```python
from build123d import *

# Parameters (mm, degrees)
F1_DEPTH = 12.7
F2_SIZE  = 6.34999
F4_D     = 22


# Not quite as in the source:
# - a fillet or chamfer is up to 0.001 mm smaller than in the source, because OpenCascade refuses the exact size


with BuildPart() as f1:
    # F0 (on Right) → F1 (new body)
    with BuildSketch(Plane.YZ):
        Polygon((0, 56.2922134995), (-25.5191382021, 25.3690239042), (-54.6409785748, 0), (-25.5191382021, -25.6692506373), (0, -56.8926632404), (25.2189133316, -25.6692506373), (54.9412034452, 0), (25.5191363394, 24.768576026), align=None)
    extrude(amount=F1_DEPTH)

    # F2 (size 6.35 in the source; OpenCascade refuses exactly that, so slightly less here)
    f2_edges = [f1.edges().sort_by_distance(p)[0] for p in [
        (12.7, -40.080058, 12.684512),
        (0, -40.080058, 12.684512),
        (12.7, -40.080058, -12.834625),
        (0, -40.080058, -12.834625),
        (12.7, -12.759569, -41.280957),
        (0, -12.759569, -41.280957),
        (0, 12.609457, -41.280957),
        (12.7, 12.609457, -41.280957),
        (0, 40.080058, -12.834625),
        (12.7, 40.080058, -12.834625),
        (12.7, 40.23017, 12.384288),
        (0, 40.23017, 12.384288),
        (0, 12.759568, 40.530395),
        (12.7, 12.759568, 40.530395),
        (0, -12.759569, 40.830619),
        (12.7, -12.759569, 40.830619),
    ]]
    chamfer(f2_edges, length=F2_SIZE)

    # F4 (through all)
    with Locations(Plane(origin=(0, 0, 0), x_dir=(0, 1, 0), z_dir=(-1, 0, 0))):
        with Locations((0, 0)):
            Hole(F4_D / 2)


solid = f1.part
```
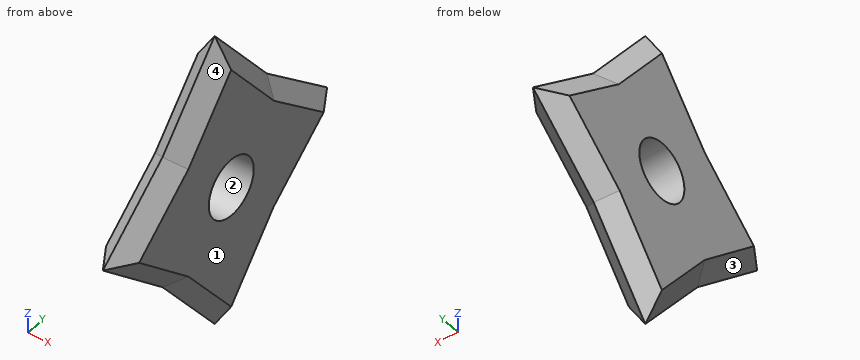
Part model, mm, in its own coordinate system. Face numbers are marked on the shaded views. Round coordinates to 2 decimals unless told otherwise and drop trailing zeros. Write each loop counter-clockwise with the first axis right and the second up, starting at its lowest first coordinate (ties: lowest second). Pieces come first, ordered by that corner, then holes. Notation, with made-up numbers: (-27.75, -2) -> (14.25, -2) arc R22 cw to (14.25, 35) -> close; hole circle Ø1 at (-29.5, 45.5). An arc over 180 degrees is marked (long way). Return JSON: item names as keys, results as strings. Group by question number.
Q1. Saw through at C-C on x = 1.75. Write the cut outline in (y, z), plus the area to 3 significant figures.
Q2. Mould opens along Z. For the marked faces 1, 2, 3 and 4 say: pulls with the +Z half, pulls with the -Z half, needs draft (parallel to the pull), parting line crosses it, or undercut.
Q3. Probe L1, parallel to Y at x = 9.5, z = -6; L2, parallel to Z at x = 6.5, y = 5; L3, parallel to Y at x = 1.25, z = -6. List the from-to ranges inside material, lowest first. Write a range as [from, to].
Q4. Pin check, flat tips, straight feed: pin 1 (1.5 mm diameter, centred on x = 3, y = -0.5, fed in from -Z); pin 2 (13 mm diameter, centred on y = 0, z = 0, fed in from +X); pin 3 (3 mm diameter, centred on x = 10, y = -25.5, fed in from +Z); pin 4 (6 mm diameter, centred on x = 10.5, y = 5.5, fed in from -Z). Stop position of each tip, or through.
Answer:
{
 "1": {"outline": "(-47.66, -0.02) -> (-22.2, -22.47) -> (-0.02, -49.6) -> (21.9, -22.46) -> (47.85, -0.04) -> (22.22, 21.53) -> (-0.03, 49.02) -> (-22.21, 22.15) -> close; hole circle Ø22 at (0, 0)", "area": "3,920 mm2"},
 "2": {"face 1": "needs draft", "face 2": "undercut", "face 3": "pulls with the -Z half", "face 4": "pulls with the +Z half"},
 "3": {"L1": "[-43.07, -9.22], [9.22, 43.17]", "L2": "[-50.46, -9.8], [9.8, 49.88]", "L3": "[-40.12, -9.22], [9.22, 40.19]"},
 "4": {"pin 1": "z = -52.49", "pin 2": "through", "pin 3": "z = 22.93", "pin 4": "z = -49.53"}
}
